Source: three-view drawing plus pictorial views. Frame: mm from the lowest corner of the part. A direction names the side the tool comes from. Coordinates: 2 decimals unless noted, no trailing zeros. Order: outer loops, then holes, each group sorted by start corner. A loop starts at its lowest first (then second) coordinate and runs counter-clockwise, first axis right, second up. Notation, with made-up numbers: (41.25, 65) -> (63.25, 65) arc R20 cw to (63.25, 71) -> close; hole circle Ø3 at (28.5, 70). An arc over 180 degrees is marked (long way). One line per question, with ' | ' between items.
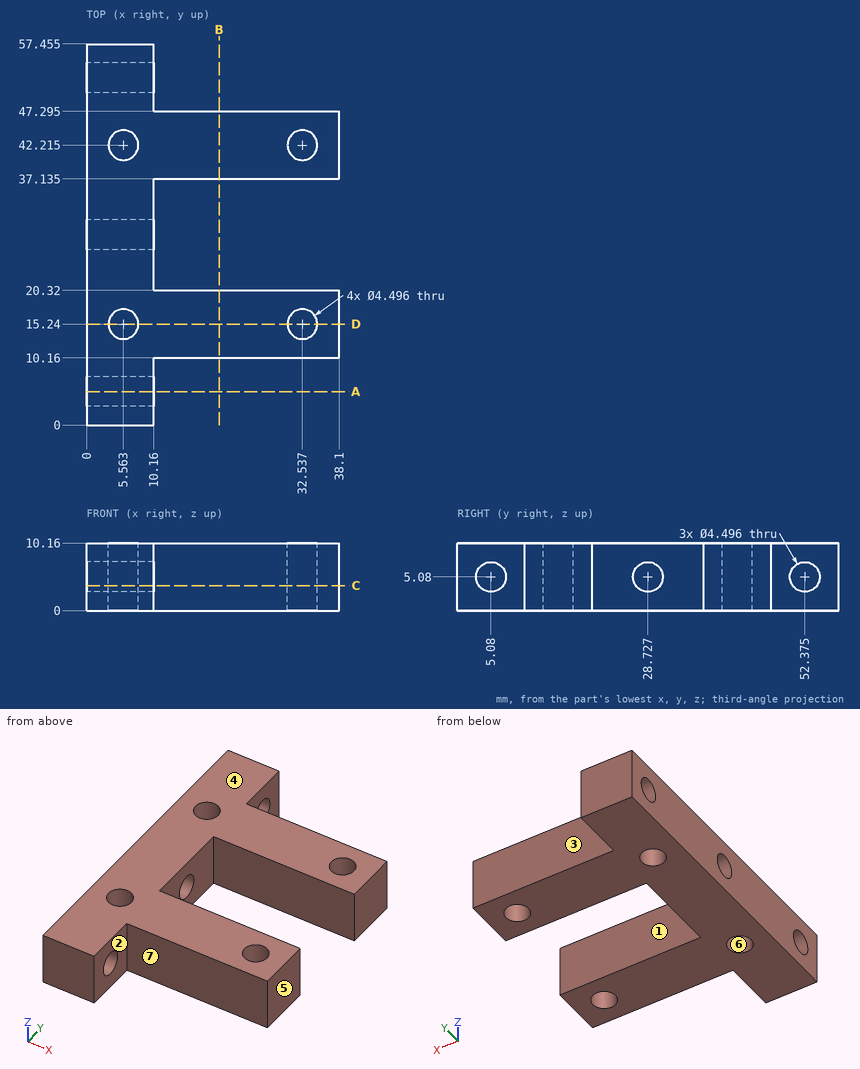
1. Mould query, pull axis Y, two halves, no side actions, for the marked faces 5, 6 and 7. Classes: released by +Y, released by -Y, zero draft, split by the parting line, or undercut.
Recorded:
face 5: zero draft | face 6: undercut | face 7: released by -Y
2. Pin query (flat end, axial travel): pin 1 Ø5 at (x, z) = (24, 6.5) entering from -Y; pin 2 Ø3 at (y, z) = (50.5, 3) entering from +X; pin 3 Ø5 at (x, z) = (21, 4.5) entering from +Y (1 decimal). Return the tip coordinate at first contact, or that it passes through.
Recorded:
pin 1: stops at y = 10.16 | pin 2: stops at x = 10.16 | pin 3: stops at y = 47.3
3. Ray query, line 1 (X direction, y = 41, z = 7.5) (1 decimal); line 2 (Y direction, x = 28, z = 8.5) (1 decimal); line 3 (Y direction, x = 7, z = 5.75) (1 decimal). Return the intervals inside material, ascending. Write a range as [from, to].
Recorded:
line 1: x = [0, 3.7], [7.5, 30.6], [34.4, 38.1] | line 2: y = [10.2, 20.3], [37.1, 47.3] | line 3: y = [0, 2.9], [7.2, 13.5], [17, 26.6], [30.9, 40.5], [43.9, 50.2], [54.5, 57.5]
4. Access query for the marked faces 1, 2, 3 and 4. Directions: +Z, -Z, +X, -X, +Y, -Y. A direction counts if a zero-diameter tool reaches every point of the face in a straight line with its end or side. Return the directions, or none.
Recorded:
face 1: +Z, -Z, +X | face 2: +Z, -Z, +X, -Y | face 3: +Z, -Z, +X, +Y | face 4: +Z, +X, -X, +Y, -Y
5. Cut plane C-C, the plane z = 3.75. Return loops of the section in (x, y) (1 decimal).
Recorded:
outline: (0, 0) -> (10.2, 0) -> (10.2, 3.3) -> (0, 3.3) -> close; (0, 6.9) -> (10.2, 6.9) -> (10.2, 10.2) -> (38.1, 10.2) -> (38.1, 20.3) -> (10.2, 20.3) -> (10.2, 26.9) -> (0, 26.9) -> close; (0, 30.5) -> (10.2, 30.5) -> (10.2, 37.1) -> (38.1, 37.1) -> (38.1, 47.3) -> (10.2, 47.3) -> (10.2, 50.6) -> (0, 50.6) -> close; (0, 54.2) -> (10.2, 54.2) -> (10.2, 57.5) -> (0, 57.5) -> close; hole circle Ø4.5 at (5.6, 15.2); hole circle Ø4.5 at (5.6, 42.2); hole circle Ø4.5 at (32.5, 15.2); hole circle Ø4.5 at (32.5, 42.2)
6. Cut plane A-A, the plane y = 5.08. Return loops of the section in (x, z).
Recorded:
outline: (0, 0) -> (10.16, 0) -> (10.16, 2.83) -> (0, 2.83) -> close; (0, 7.33) -> (10.16, 7.33) -> (10.16, 10.16) -> (0, 10.16) -> close
7. Cut plane B-B, the plane x = 20. Return loops of the section in (y, z) (1 decimal).
Recorded:
outline: (10.2, 0) -> (20.3, 0) -> (20.3, 10.2) -> (10.2, 10.2) -> close; (37.1, 0) -> (47.3, 0) -> (47.3, 10.2) -> (37.1, 10.2) -> close
8. Cut plane D-D, the plane y = 15.24. Return loops of the section in (x, z) (1 decimal), and give its area (3 significant figures).
Recorded:
outline: (0, 0) -> (3.3, 0) -> (3.3, 10.2) -> (0, 10.2) -> close; (7.8, 0) -> (30.3, 0) -> (30.3, 10.2) -> (7.8, 10.2) -> close; (34.8, 0) -> (38.1, 0) -> (38.1, 10.2) -> (34.8, 10.2) -> close | area: 296 mm^2
